from build123d import *

# Parameters (mm, degrees)
SKETCH1_W           = 2300
SKETCH1_H           = 150
BOSS_EXTRUDE1_DEPTH = 100
SKETCH2_W           = 80
SKETCH2_H           = 130
CUT_EXTRUDE1_DEPTH  = 2304.394234602
FILLET1_R           = 10
FILLET2_R           = 20
SKETCH3_R           = 25
CUT_EXTRUDE2_DEPTH  = 1157.773530126
CUT_EXTRUDE3_DEPTH  = 1157.773530126


with BuildPart() as part:
    # Sketch1 → Boss-Extrude1 (new body)
    with BuildSketch(Plane.XY):
        Rectangle(SKETCH1_W, SKETCH1_H)
    extrude(amount=BOSS_EXTRUDE1_DEPTH)

    # Sketch2 → Cut-Extrude1 (cut, through all)
    with BuildSketch(Plane(origin=(1150, 0, 0), x_dir=(0, 0, -1), z_dir=(1, 0, 0))):
        with Locations((-50, 0)):
            Rectangle(SKETCH2_W, SKETCH2_H)
    extrude(amount=-CUT_EXTRUDE1_DEPTH, mode=Mode.SUBTRACT)

    # Fillet1
    fillet1_edges = [part.edges().sort_by_distance(p)[0] for p in [
        (0, 65, 90),
        (0, 65, 10),
        (0, -65, 10),
        (0, -65, 90),
    ]]
    fillet(fillet1_edges, radius=FILLET1_R)

    # Fillet2
    fillet2_edges = [part.edges().sort_by_distance(p)[0] for p in [
        (0, -75, 100),
        (0, -75, 0),
        (0, 75, 0),
        (0, 75, 100),
    ]]
    fillet(fillet2_edges, radius=FILLET2_R)

    # Sketch3 → Cut-Extrude2 (cut, through all)
    with BuildSketch(Plane(origin=(0, 0, 0), x_dir=(-1, 0, 0), z_dir=(0, 0, -1))):
        Circle(SKETCH3_R)
        with Locations((-1098.86, 0)):
            Circle(SKETCH3_R)
        with Locations((1098.86, 0)):
            Circle(SKETCH3_R)
    extrude(amount=-CUT_EXTRUDE2_DEPTH, mode=Mode.SUBTRACT)

    # Sketch4 → Cut-Extrude3 (cut, through all)
    with BuildSketch(Plane(origin=(0, 0, 0), x_dir=(-1, 0, 0), z_dir=(0, 0, -1))):
        with BuildLine():
            Line((-799.995, 12.91), (-702.465, 12.91))
            ThreePointArc((-702.465, 12.91), (-689.555, 0), (-702.465, -12.91))
            Line((-702.465, -12.91), (-799.995, -12.91))
            ThreePointArc((-799.995, -12.91), (-812.905, 0), (-799.995, 12.91))
        make_face()
        with BuildLine():
            Line((799.995, 12.91), (702.465, 12.91))
            ThreePointArc((702.465, 12.91), (689.555, 0), (702.465, -12.91))
            Line((702.465, -12.91), (799.995, -12.91))
            ThreePointArc((799.995, -12.91), (812.905, 0), (799.995, 12.91))
        make_face()
    extrude(amount=-CUT_EXTRUDE3_DEPTH, mode=Mode.SUBTRACT)


solid = part.part
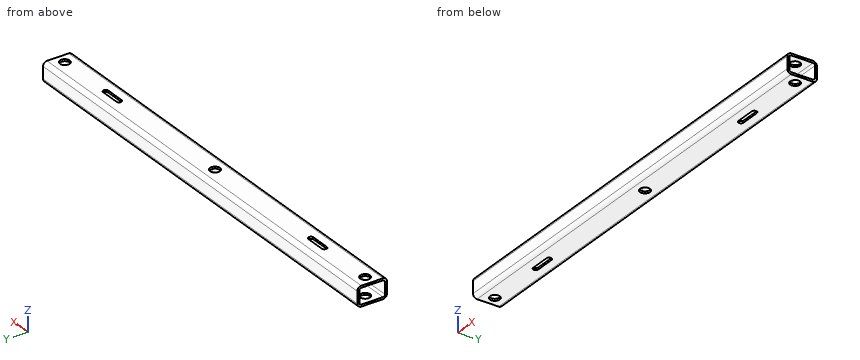
Geometry: final body of the model. Coordinates: model frame, mm. Give positions to 0.01 mm unless a question says otherwise; leave off trailing zeros. Write each loop counter-clockwise with the first axis right and the second up, starting at its lowest first coordinate (ties: lowest second). Pieces come first, ordered by that corner, then holes.
(1) Ray query, line 1 (Z direction, x = 918, y = -33.5); line 2 (Y direction, x = 145.5, z = 57.5); line 3 (Z direction, x = -245, y = 57). Return the intervals inside material, ascending.
(2) Cut plane B-B, the plane x = 1098.86. Return loops of the section in (y, z), then the cut area to 3 significant figures.
(3) Cut plane A-A, the plane z = 40.5. Return loops of the section in (x, y), then the cut area to 3 significant figures.
(4) Cut plane C-C, the plane x = 386.5. Return loops of the section in (y, z), then the cut area to 3 significant figures.
(5) First-contact query: P1, Ø3, axis at x = -742, z = 3.5, coming from the +Y side; P2, Ø5, axis at x = -770, z = 92.5, coming from the +Y side; P3, Ø8, axis at x = 743, z = 96, coming from the +Y side. Flat tips, straight axial feed; report the tip coordinate or a pass-through.
Values follow:
1. line 1: z = 0 to 10, 90 to 100
1. line 2: y = -75 to -65, 65 to 75
1. line 3: z = 0.1 to 10.2, 89.8 to 99.9
2. outline: (-75, 20) arc R20 ccw to (-55, 0) - (-25, 0) - (-25, 10) - (-55, 10) arc R10 cw to (-65, 20) - (-65, 80) arc R10 cw to (-55, 90) - (-25, 90) - (-25, 100) - (-55, 100) arc R20 ccw to (-75, 80) - close; (25, 0) - (55, 0) arc R20 ccw to (75, 20) - (75, 80) arc R20 ccw to (55, 100) - (25, 100) - (25, 90) - (55, 90) arc R10 cw to (65, 80) - (65, 20) arc R10 cw to (55, 10) - (25, 10) - close
2. area: 3,340 mm2
3. outline: (-1150, -75) - (1150, -75) - (1150, -65) - (-1150, -65) - close; (-1150, 65) - (1150, 65) - (1150, 75) - (-1150, 75) - close
3. area: 46,000 mm2
4. outline: (-75, 20) arc R20 ccw to (-55, 0) - (55, 0) arc R20 ccw to (75, 20) - (75, 80) arc R20 ccw to (55, 100) - (-55, 100) arc R20 ccw to (-75, 80) - close; hole (-65, 20) arc R10 ccw to (-55, 10) - (55, 10) arc R10 ccw to (65, 20) - (65, 80) arc R10 ccw to (55, 90) - (-55, 90) arc R10 ccw to (-65, 80) - close
4. area: 4,340 mm2
5. P1: stops at y = 68.23
5. P2: stops at y = 72.32
5. P3: stops at y = 71
